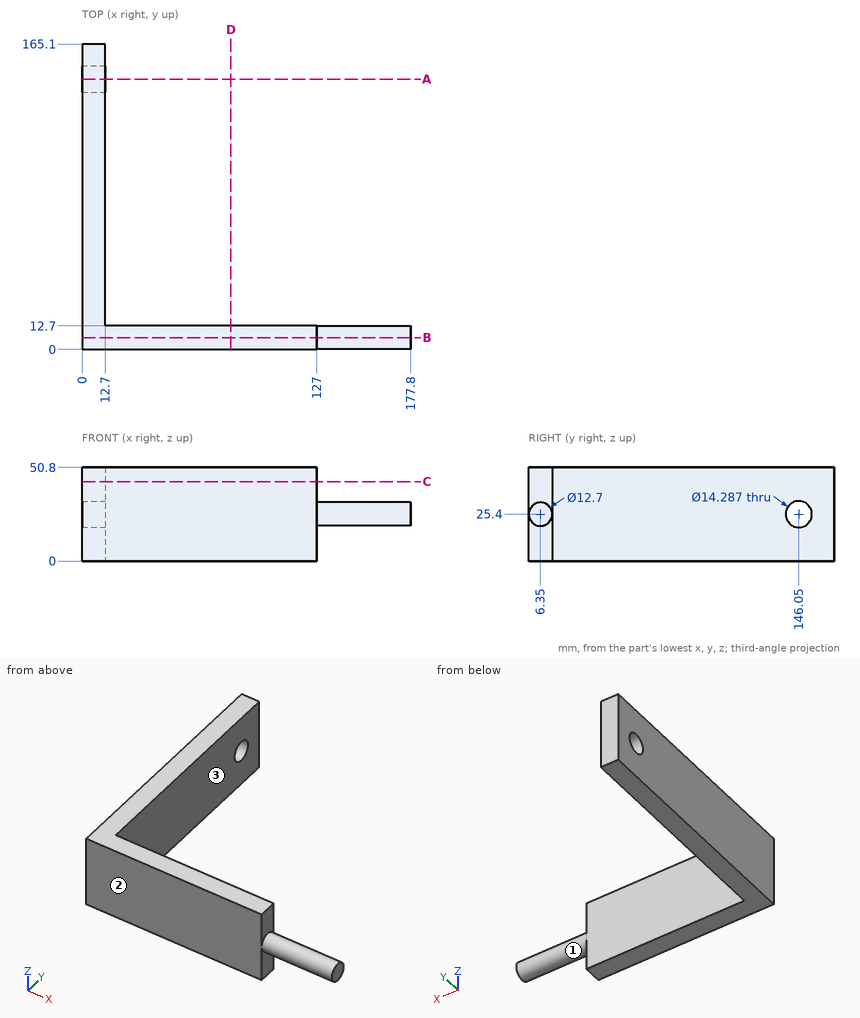
Here's the drawing with two shaded views (mm, measured from the low corner). I have some questions. A direction names the side the tool comes from. Coordinates: 2 decimals unless noted, no trailing zeros. Order: outer loops, then holes, each group sorted by start corner. A loop starts at its lowest first (then second) coordinate and runs counter-clockwise, first axis right, second up.
Q1. Suppose I cut it at D-D on x = 80.5. Please give me the cut outline in (y, z), and give its area (3 significant figures).
Q2. Please list where these lines run through material, in increasing order: L1, parallel to Y at x = 3, z = 25; L2, parallel to Z at x = 8.5, y = 146.05; L3, parallel to X at y = 85.5, z = 33.5.
Q3. Suppose I cut it at C-C on z = 43. Please give me the cut outline in (x, y).
Q4. Suppose I cut it at A-A on y = 146.05. Please give me the cut outline in (x, z), and give its area (3 significant figures).
Q5. Will these pins go through, and if not, where does the flat tip stop? pin 1 (1.5 mm diameter, centred on x = 71, z = 44.5, fed in from +Y); pin 2 (15 mm diameter, centred on y = 105.5, z = 20, fed in from +X); pin 3 (6.5 mm diameter, centred on y = 5.5, z = 38.5, fed in from +X).
Q6. Which directions (+Z, -Z, +X, -X, +Y, -Y) give clear straight access to the entire face, cutting with the end or side of a thin tool? Please do the marked faces 1, 2 and 3.
Q7. Suppose I cut it at B-B on y = 6.35. Please give me the cut outline in (x, z).
Answer:
1. outline: (0, 0) - (12.7, 0) - (12.7, 50.8) - (0, 50.8) - close
1. area: 645 mm2
2. L1: y = 0 to 138.92, 153.18 to 165.1
2. L2: z = 0 to 18.26, 32.54 to 50.8
2. L3: x = 0 to 12.7
3. outline: (0, 0) - (127, 0) - (127, 12.7) - (12.7, 12.7) - (12.7, 165.1) - (0, 165.1) - close
4. outline: (0, 0) - (12.7, 0) - (12.7, 18.26) - (0, 18.26) - close; (0, 32.54) - (12.7, 32.54) - (12.7, 50.8) - (0, 50.8) - close
4. area: 464 mm2
5. pin 1: stops at y = 12.7
5. pin 2: stops at x = 12.7
5. pin 3: stops at x = 127
6. face 1: +X
6. face 2: +Z, -Z, +X, -X, -Y
6. face 3: +Z, -Z, +X, +Y
7. outline: (0, 0) - (127, 0) - (127, 19.05) - (177.8, 19.05) - (177.8, 31.75) - (127, 31.75) - (127, 50.8) - (0, 50.8) - close
